The listing builds one solid part. Answer for the finished solid, in the listing's coordinates (mm). Face numbers are marked on the shaded views. A direction names the side the tool comes from. Coordinates: 2 decimals unless noted, no trailing zeros. Write each loop counter-clockwise with the first axis right and the second up, starting at its lowest first coordinate (ties: lowest second). Pieces come first, ordered by that corner, then holes.
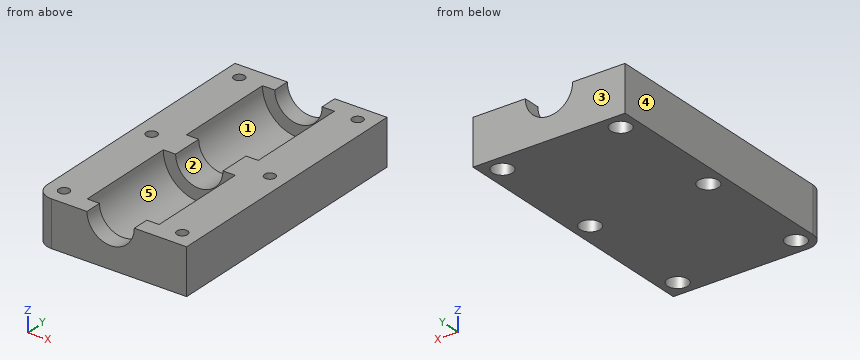
```python
from build123d import *

# Parameters (mm, degrees)
PAD_DEPTH       = 80
SKETCH001_R     = 1.6
POCKET_DEPTH    = 13.501
SKETCH002_R     = 3
POCKET001_DEPTH = 5
SKETCH003_R     = 10.65
POCKET002_DEPTH = 30.4
SKETCH004_R     = 10.65
POCKET003_DEPTH = 30.4
FILLET_R        = 5


with BuildPart() as part:
    # Sketch → Pad (new body)
    with BuildSketch(Plane.XZ):
        with BuildLine():
            Line((22.5, 0), (22.5, -13.5))
            Line((22.5, -13.5), (-22.5, -13.5))
            Line((-22.5, -13.5), (-22.5, 0))
            Line((-22.5, 0), (-7, 0))
            ThreePointArc((-7, 0), (0, -7), (7, 0))
            Line((7, 0), (22.5, 0))
        make_face()
    extrude(amount=PAD_DEPTH)

    # Sketch001 → Pocket (cut, through all)
    with BuildSketch(Plane.XY):
        with Locations((-17.5, -5)):
            Circle(SKETCH001_R)
        with Locations((-17.5, -40)):
            Circle(SKETCH001_R)
        with Locations((-17.5, -75)):
            Circle(SKETCH001_R)
        with Locations((17.5, -5)):
            Circle(SKETCH001_R)
        with Locations((17.5, -40)):
            Circle(SKETCH001_R)
        with Locations((17.5, -75)):
            Circle(SKETCH001_R)
    extrude(amount=-POCKET_DEPTH, mode=Mode.SUBTRACT)

    # Sketch002 (on DatumPlane) → Pocket001 (cut)
    with BuildSketch(Plane.XY.offset(-13.5)):
        with Locations((-17.5, -5)):
            Circle(SKETCH002_R)
        with Locations((-17.5, -40)):
            Circle(SKETCH002_R)
        with Locations((-17.5, -75)):
            Circle(SKETCH002_R)
        with Locations((17.5, -5)):
            Circle(SKETCH002_R)
        with Locations((17.5, -40)):
            Circle(SKETCH002_R)
        with Locations((17.5, -75)):
            Circle(SKETCH002_R)
    extrude(amount=POCKET001_DEPTH, mode=Mode.SUBTRACT)

    # Sketch003 (on DatumPlane) → Pocket002 (cut)
    with BuildSketch(Plane.XZ.offset(5)):
        Circle(SKETCH003_R)
    extrude(amount=POCKET002_DEPTH, mode=Mode.SUBTRACT)

    # Sketch004 (on DatumPlane) → Pocket003 (cut)
    with BuildSketch(Plane.XZ.offset(75)):
        Circle(SKETCH004_R)
    extrude(amount=-POCKET003_DEPTH, mode=Mode.SUBTRACT)

    # Fillet
    fillet_edges = [part.edges().sort_by_distance(p)[0] for p in [
        (-22.5, -80, -6.75),
    ]]
    fillet(fillet_edges, radius=FILLET_R)


solid = part.part
```
(1) Section B-B, the plane y = -40 is taken. Write down the section's boundary in (x, z).
(2) For a pull along Y with two mould halves and no side action, classify the marked faces 3, 4 and 5 as pulls with the +Y half, pulls with the -Y half, needs draft (parallel to the pull), parting line crosses it, or undercut.
(3) Each of these flat-tipped pins is pushed along its axis until it touches: pin 1 (1.9 mm diameter, centred on x = 17.5, y = -75, fed in from +Z); pin 2 (5.5 mm diameter, centred on x = 17.5, y = -5, fed in from -Z); pin 3 (5 mm diameter, centred on x = -0.5, y = -33.5, fed in from +Z). Where does it stop, or does it pass through?
(4) Find the intervals of material crossed by probe 1 along Y at (x, z) = (-17.5, -10.5); probe 2 along Y at (x, z) = (4.5, -8); probe 3 along Y at (x, z) = (-17.5, -3), in increasing order.
(5) Section D-D, the plane z = -12.25 is taken. Write down the section's boundary in (x, y).
(6) Section C-C, the plane x = 17.5 is taken. Write down the section's boundary in (y, z).
(7) Which of the six approach directions +Z, -Z, +X, -X, +Y, -Y give full straight-line access (tool end or side, diameter ignored) to the marked faces 1 and 2?
(8) Section A-A, the plane z = -1.5 is taken. State how many separate pieces and enclosed holes the cut face has, plus the area to 3 significant figures.
Solution:
1. outline: (-22.5, -13.5) - (-20.5, -13.5) - (-20.5, -8.5) - (-19.1, -8.5) - (-19.1, 0) - (-22.5, 0) - close; (-15.9, -8.5) - (-14.5, -8.5) - (-14.5, -13.5) - (14.5, -13.5) - (14.5, -8.5) - (15.9, -8.5) - (15.9, 0) - (7, 0) arc R7 cw to (-7, 0) - (-15.9, 0) - close; (19.1, -8.5) - (20.5, -8.5) - (20.5, -13.5) - (22.5, -13.5) - (22.5, 0) - (19.1, 0) - close
2. face 3: pulls with the +Y half
2. face 4: needs draft
2. face 5: undercut
3. pin 1: passes through
3. pin 2: stops at z = -8.5
3. pin 3: stops at z = -6.67
4. probe 1: y = -80 to -78, -72 to -43, -37 to -8, -2 to 0
4. probe 2: y = -80 to -75, -44.6 to -35.4, -5 to 0
4. probe 3: y = -80 to -76.6, -73.4 to -41.6, -38.4 to -6.6, -3.4 to 0
5. outline: (-22.5, -75) arc R5 ccw to (-17.5, -80) - (22.5, -80) - (22.5, 0) - (-22.5, 0) - close; hole circle Ø6 at (-17.5, -75); hole circle Ø6 at (-17.5, -40); hole circle Ø6 at (-17.5, -5); hole circle Ø6 at (17.5, -75); hole circle Ø6 at (17.5, -40); hole circle Ø6 at (17.5, -5)
6. outline: (-80, -13.5) - (-78, -13.5) - (-78, -8.5) - (-76.6, -8.5) - (-76.6, 0) - (-80, 0) - close; (-73.4, -8.5) - (-72, -8.5) - (-72, -13.5) - (-43, -13.5) - (-43, -8.5) - (-41.6, -8.5) - (-41.6, 0) - (-73.4, 0) - close; (-38.4, -8.5) - (-37, -8.5) - (-37, -13.5) - (-8, -13.5) - (-8, -8.5) - (-6.6, -8.5) - (-6.6, 0) - (-38.4, 0) - close; (-3.4, -8.5) - (-2, -8.5) - (-2, -13.5) - (0, -13.5) - (0, 0) - (-3.4, 0) - close
7. face 1: +Z
7. face 2: +Z, +Y, -Y
8. separate pieces: 2
8. enclosed holes: 6
8. area: 2,000 mm2
